```python
from build123d import *

# Parameters (mm, degrees)
SKETCH_1_W               = 25
SKETCH_1_H               = 58
EXTRUDE_1_DEPTH          = 4
SKETCH_2_R               = 1.525
CUT_EXTRUDE_1_DEPTH      = 1
CUT_EXTRUDE_1_DEPTH_BACK = 5
FILLET_1_R               = 3
CUT_EXTRUDE_2_DEPTH      = 1
CUT_EXTRUDE_2_DEPTH_BACK = 5


with BuildPart() as part:
    # 草图1 → 凸台-拉伸1 (new body)
    with BuildSketch(Plane.XY):
        Rectangle(SKETCH_1_W, SKETCH_1_H)
    extrude(amount=EXTRUDE_1_DEPTH)

    # 草图2 → 切除-拉伸1 (cut, two sides)
    with BuildSketch(Plane(origin=(0, 0, 0), x_dir=(-1, 0, 0), z_dir=(0, 0, -1))) as cut_extrude_1_sk:
        with Locations((0, 24.999999999)):
            Circle(SKETCH_2_R)
        with Locations((0, -5.000000001)):
            Circle(SKETCH_2_R)
    extrude(amount=CUT_EXTRUDE_1_DEPTH, mode=Mode.SUBTRACT)
    extrude(cut_extrude_1_sk.sketch, amount=-CUT_EXTRUDE_1_DEPTH_BACK, mode=Mode.SUBTRACT)

    # 圆角1
    fillet_1_edges = [part.edges().sort_by_distance(p)[0] for p in [
        (12.5, -29, 2),
        (-12.5, -29, 2),
        (-12.5, 29, 2),
        (12.5, 29, 2),
    ]]
    fillet(fillet_1_edges, radius=FILLET_1_R)

    # 草图3 → 切除-拉伸2 (cut, two sides)
    with BuildSketch(Plane.XY.offset(4)) as cut_extrude_2_sk:
        with BuildLine():
            Line((5, 15.999999999), (5, 3.999999999))
            ThreePointArc((5, 3.999999999), (0, -1.000000001), (-5, 3.999999999))
            Line((-5, 3.999999999), (-5, 15.999999999))
            ThreePointArc((-5, 15.999999999), (0, 20.999999999), (5, 15.999999999))
        make_face()
        with BuildLine():
            Line((5, -14), (5, -20))
            ThreePointArc((5, -20), (0, -25), (-5, -20))
            Line((-5, -20), (-5, -14))
            ThreePointArc((-5, -14), (0, -9), (5, -14))
        make_face()
    extrude(amount=CUT_EXTRUDE_2_DEPTH, mode=Mode.SUBTRACT)
    extrude(cut_extrude_2_sk.sketch, amount=-CUT_EXTRUDE_2_DEPTH_BACK, mode=Mode.SUBTRACT)


solid = part.part
```
The model under review builds one solid part; all positions refer to its coordinate system, in mm. A direction names the side the tool comes from. Round coordinates to 2 decimals unless told otherwise and drop trailing zeros. Order: outer loops, then holes, each group sorted by start corner. A loop starts at its lowest first (then second) coordinate and runs counter-clockwise, first axis right, second up. Notation, with made-up numbers: (32.5, -10.5) -> (58.5, -10.5) arc R19 cw to (58.5, 25.5) -> close; hole circle Ø2 at (-20.75, 89). An arc over 180 degrees is marked (long way). Use a Markdown table: item, result.
Q1. We need section C-C on x = 3. Write out the cut boundary in (y, z).
Values:
| item | result |
|---|---|
| outline | (-29, 0) -> (-24, 0) -> (-24, 4) -> (-29, 4) -> close; (-10, 0) -> (0, 0) -> (0, 4) -> (-10, 4) -> close; (20, 0) -> (29, 0) -> (29, 4) -> (20, 4) -> close |
Q2. We need section B-B on z = 1. Write out the cut boundary in (x, y) (3 decimals).
Values:
| item | result |
|---|---|
| outline | (-12.5, -26) arc R3 ccw to (-9.5, -29) -> (9.5, -29) arc R3 ccw to (12.5, -26) -> (12.5, 26) arc R3 ccw to (9.5, 29) -> (-9.5, 29) arc R3 ccw to (-12.5, 26) -> close; hole (-5, -20) arc R5 ccw to (5, -20) -> (5, -14) arc R5 ccw to (-5, -14) -> close; hole (-5, 4) arc R5 ccw to (5, 4) -> (5, 16) arc R5 ccw to (-5, 16) -> close; hole circle Ø3.05 at (0, -5); hole circle Ø3.05 at (0, 25) |
Q3. We need section D-D on y = 11.5. Write out the cut boundary in (x, z), then the cut area to 3 significant figures.
Values:
| item | result |
|---|---|
| outline | (-12.5, 0) -> (-5, 0) -> (-5, 4) -> (-12.5, 4) -> close; (5, 0) -> (12.5, 0) -> (12.5, 4) -> (5, 4) -> close |
| area | 60.0 mm^2 |
Q4. We need section A-A on y = 25. Write out the cut boundary in (x, z) (3 decimals), then the cut area to 3 significant figures.
Values:
| item | result |
|---|---|
| outline | (-12.5, 0) -> (-1.525, 0) -> (-1.525, 4) -> (-12.5, 4) -> close; (1.525, 0) -> (12.5, 0) -> (12.5, 4) -> (1.525, 4) -> close |
| area | 87.8 mm^2 |
Q5. Tool access review of faces 1 (the flat face through (-5, 10, 2)), 2 (the cylindrical face through (-11.64, -28.1, 2.03)): name each direction out of +Z, -Z, +X, -X, +Y, -Y from which nothing blocks a thin tool from reaching the whole face with its end or side.
Values:
| item | result |
|---|---|
| face 1 | +Z, -Z |
| face 2 | +Z, -Z, -X, -Y |
Q6. For line 1 (Y direction, x = 0, z = 0.85) (3 decimals); line 2 (X direction, y = 13.5, z = 3); line 3 (X direction, y = 25, z = 3.25) (3 decimals), list the stretches that pass through material, from the lowest coordinate up.
Values:
| item | result |
|---|---|
| line 1 | y = -29 to -25, -9 to -6.525, -3.475 to -1, 21 to 23.475, 26.525 to 29 |
| line 2 | x = -12.5 to -5, 5 to 12.5 |
| line 3 | x = -12.5 to -1.525, 1.525 to 12.5 |
